```python
from build123d import *

# Parameters (mm, degrees)
SKETCH2_W           = 120
SKETCH2_H           = 100
BOSS_EXTRUDE1_DEPTH = 2.5
SKETCH3_R           = 1.5
CUT_EXTRUDE1_DEPTH  = 5
SKETCH4_R           = 5
CUT_EXTRUDE2_DEPTH  = 5
CUT_EXTRUDE3_DEPTH  = 10
SKETCH6_W           = 10
SKETCH6_H           = 5
SKETCH6_W_2         = 5
SKETCH6_H_2         = 10
BOSS_EXTRUDE2_DEPTH = 15
SKETCH7_R           = 1.5
CUT_EXTRUDE4_DEPTH  = 82.946628973
SKETCH8_R           = 1.5
CUT_EXTRUDE5_DEPTH  = 99.001275502
FILLET1_R           = 2
SKETCH9_W           = 10
SKETCH9_H           = 5
SKETCH9_W_2         = 5
SKETCH9_H_2         = 10
CUT_EXTRUDE6_DEPTH  = 15


with BuildPart() as part:
    # Sketch2 → Boss-Extrude1 (new body)
    with BuildSketch(Plane(origin=(0, 0, 0), x_dir=(1, 0, 0), z_dir=(0, 1, 0))):
        Rectangle(SKETCH2_W, SKETCH2_H)
    extrude(amount=BOSS_EXTRUDE1_DEPTH)

    # Sketch3 → Cut-Extrude1 (cut)
    with BuildSketch(Plane(origin=(0, 2.5, 0), x_dir=(1, 0, 0), z_dir=(0, 1, 0))):
        with Locations(Location((-55, 45, 0), (0, 0, 270))):
            Circle(SKETCH3_R)
        with Locations(Location((55, 45, 0), (0, 0, 270))):
            Circle(SKETCH3_R)
        with Locations(Location((55, -45, 0), (0, 0, 270))):
            Circle(SKETCH3_R)
        with Locations(Location((-55, -45, 0), (0, 0, 270))):
            Circle(SKETCH3_R)
    extrude(amount=-CUT_EXTRUDE1_DEPTH, mode=Mode.SUBTRACT)

    # Sketch4 → Cut-Extrude2 (cut)
    with BuildSketch(Plane(origin=(0, 2.5, 0), x_dir=(1, 0, 0), z_dir=(0, 1, 0))):
        with Locations(Location((-38, 28, 0), (0, 0, 270))):
            Circle(SKETCH4_R)
        with Locations(Location((-4, 28, 0), (0, 0, 270))):
            Circle(SKETCH4_R)
        with Locations(Location((38, 6, 0), (0, 0, 270))):
            Circle(SKETCH4_R)
        with Locations(Location((38, -28, 0), (0, 0, 270))):
            Circle(SKETCH4_R)
    extrude(amount=-CUT_EXTRUDE2_DEPTH, mode=Mode.SUBTRACT)

    # Sketch5 → Cut-Extrude3 (cut)
    with BuildSketch(Plane(origin=(0, 2.5, 0), x_dir=(1, 0, 0), z_dir=(0, 1, 0))):
        with BuildLine():
            Line((-4, 33), (2, 33))
            ThreePointArc((2, 33), (7, 28), (2, 23))
            Line((2, 23), (-4, 23))
            ThreePointArc((-4, 23), (-9, 28), (-4, 33))
        make_face()
        with BuildLine():
            Line((33, 6), (33, 12))
            ThreePointArc((33, 12), (38, 17), (43, 12))
            Line((43, 12), (43, 6))
            ThreePointArc((43, 6), (38, 1), (33, 6))
        make_face()
    extrude(amount=-CUT_EXTRUDE3_DEPTH, mode=Mode.SUBTRACT)

    # Sketch6 → Boss-Extrude2 (add)
    with BuildSketch(Plane(origin=(0, 2.5, 0), x_dir=(1, 0, 0), z_dir=(0, 1, 0))):
        with Locations((-21, 5.5)):
            Rectangle(SKETCH6_W, SKETCH6_H)
        with Locations((57.5, -11)):
            Rectangle(SKETCH6_W_2, SKETCH6_H_2)
        with Locations((-21, 47.5)):
            Rectangle(SKETCH6_W, SKETCH6_H)
        with Locations((15.5, -11)):
            Rectangle(SKETCH6_W_2, SKETCH6_H_2)
    extrude(amount=BOSS_EXTRUDE2_DEPTH)

    # Sketch7 → Cut-Extrude4 (cut, through all)
    with BuildSketch(Plane.XY.offset(-3)):
        with Locations((-21, 8.5)):
            Circle(SKETCH7_R)
        with BuildLine():
            Line((-16, 8.5), (-16, 17.5))
            Line((-16, 17.5), (-26, 17.5))
            Line((-26, 17.5), (-26, 8.5))
            ThreePointArc((-26, 8.5), (-21, 13.5), (-16, 8.5))
        make_face()
    extrude(amount=-CUT_EXTRUDE4_DEPTH, mode=Mode.SUBTRACT)

    # Sketch8 → Cut-Extrude5 (cut, through all)
    with BuildSketch(Plane(origin=(13, 0, -13), x_dir=(0, 0, 1), z_dir=(-1, 0, 0))):
        with Locations((24, 8.5)):
            Circle(SKETCH8_R)
        with BuildLine():
            Line((29, 8.5), (29, 17.5))
            Line((29, 17.5), (19, 17.5))
            Line((19, 17.5), (19, 8.5))
            ThreePointArc((19, 8.5), (24, 13.5), (29, 8.5))
        make_face()
    extrude(amount=-CUT_EXTRUDE5_DEPTH, mode=Mode.SUBTRACT)

    # Fillet1
    fillet1_edges = [part.edges().sort_by_distance(p)[0] for p in [
        (-22.5, 8.5, -8),
        (-22.5, 8.5, -50),
        (-22.5, 8.5, -45),
        (-22.5, 8.5, -3),
        (60, 8.5, 9.5),
        (55, 8.5, 9.5),
        (18, 8.5, 9.5),
        (13, 8.5, 9.5),
    ]]
    fillet(fillet1_edges, radius=FILLET1_R)

    # Sketch9 → Cut-Extrude6 (cut)
    with BuildSketch(Plane(origin=(0, 2.5, 0), x_dir=(1, 0, 0), z_dir=(0, 1, 0))):
        with Locations((-21, 47.5)):
            Rectangle(SKETCH9_W, SKETCH9_H)
        with Locations((15.5, -11)):
            Rectangle(SKETCH9_W_2, SKETCH9_H_2)
    extrude(amount=CUT_EXTRUDE6_DEPTH, mode=Mode.SUBTRACT)


solid = part.part
```
The model under review builds one solid part; all positions refer to its coordinate system, in mm. A direction names the side the tool comes from. Round coordinates to 2 decimals unless told otherwise and drop trailing zeros. Loops run counter-clockwise (first coordinate to the right, second up) from the corner with the lowest first, then second, coordinate; pieces in that order, holes last. Notation, with made-up numbers: (10.5, -5.5) -> (42.5, -5.5) arc R25 ccw to (42.5, 10.5) -> close; hole circle Ø6 at (54.25, -26.75). An arc over 180 degrees is marked (long way). Answer in a Markdown table with one row per item.
1) Draft analysis for pull direction X (two halves, no side actions). For faces 1 (the flat face through (-1, 1, -23)), 2 (the flat face through (60, 2, 4)), 3 (the cylindrical face through (-21.1, 13.5, -5.5)), state which applies: pulls with the +X half, pulls with the -X half, needs draft (parallel to the pull), parting line crosses it, or undercut.
Taken from the geometry:
| item | result |
|---|---|
| face 1 | undercut |
| face 2 | pulls with the +X half |
| face 3 | parting line crosses it |
2) Wall thickness on line 1 along X through (y, z) = (1.85, 45); line 2 along X through (y, z) = (1, -28.5); line 3 along X through (y, z) = (1.95, 28): over which ranges is each line inside the solid? List them lowest first.
Taken from the geometry:
| item | result |
|---|---|
| line 1 | x = -60 to -56.5, -53.5 to 53.5, 56.5 to 60 |
| line 2 | x = -60 to -42.97, -33.03 to -8.97, 6.97 to 60 |
| line 3 | x = -60 to 33, 43 to 60 |
3) Consider section C-C, the plane z = 28. Write out the cut boundary in (x, y), plus the area to 3 significant figures.
Taken from the geometry:
| item | result |
|---|---|
| outline | (-60, 0) -> (33, 0) -> (33, 2.5) -> (-60, 2.5) -> close; (43, 0) -> (60, 0) -> (60, 2.5) -> (43, 2.5) -> close |
| area | 275 mm² |
4) Consider section D-D, the plane z = -45. Write out the cut boundary in (x, y).
Taken from the geometry:
| item | result |
|---|---|
| outline | (-60, 0) -> (-56.5, 0) -> (-56.5, 2.5) -> (-60, 2.5) -> close; (-53.5, 0) -> (53.5, 0) -> (53.5, 2.5) -> (-53.5, 2.5) -> close; (56.5, 0) -> (60, 0) -> (60, 2.5) -> (56.5, 2.5) -> close |
5) Tool access review of faces 4 (the flat face through (55, 5, 13)), 5 (the flat face through (-23, 5, -3)), 6 (the flat face through (57, 5, 6)), 7 (the cylindrical face through (38, 1, -17)): name each direction out of +Z, -Z, +X, -X, +Y, -Y from which nothing blocks a thin tool from reaching the whole face with its end or side.
Taken from the geometry:
| item | result |
|---|---|
| face 4 | +Z, -Z, -X, +Y |
| face 5 | +Z, +X, -X, +Y |
| face 6 | -Z, +X, -X, +Y |
| face 7 | +Y, -Y |
6) Consider section A-A, the plane x = -21. Write out the cut boundary in (y, z).
Taken from the geometry:
| item | result |
|---|---|
| outline | (0, -50) -> (2.5, -50) -> (2.5, -8) -> (5, -8) arc R2 ccw to (7, -6) -> (7, -5) arc R2 ccw to (5, -3) -> (2.5, -3) -> (2.5, 50) -> (0, 50) -> close; (10, -6) arc R2 ccw to (12, -8) -> (13.5, -8) -> (13.5, -3) -> (12, -3) arc R2 ccw to (10, -5) -> close |
7) Consider section B-B, the plane x = 35. Write out the cut boundary in (y, z), plus the area to 3 significant figures.
Taken from the geometry:
| item | result |
|---|---|
| outline | (0, -50) -> (2.5, -50) -> (2.5, -16) -> (0, -16) -> close; (0, -2) -> (2.5, -2) -> (2.5, 24) -> (0, 24) -> close; (0, 32) -> (2.5, 32) -> (2.5, 50) -> (0, 50) -> close |
| area | 195 mm² |
8) For pin 1 Ø12 at (x, z) = (44, -5.5) entering from +Y; pin 2 Ø1.5 at (y, z) = (5.5, -4.5) entering from +X; pin 3 Ø8 at (x, z) = (-47, 32) entering from -Y; pin 4 Ø1.5 at (x, y) = (56.5, 7) entering from +Z, all flat-tipped, find the tip position at first contact; note any pin that passes through.
Taken from the geometry:
| item | result |
|---|---|
| pin 1 | stops at y = 2.5 |
| pin 2 | stops at x = -16 |
| pin 3 | stops at y = 0 |
| pin 4 | stops at z = 16 |
